Input: dimensioned drawing with shaded views. Units: mm. Origin: part minimum x, y, z. A direction names the side the tool comes from. Round coordinates to 2 decimals unless told otherwise and drop trailing zeros. Write each loop counter-clockwise with the first axis right and the second up, starting at its lowest first coordinate (ties: lowest second). Pieces come first, ordered by that corner, then holes. Notation, with made-up numbers: M 62.5,29.5 L 70.5,29.5 A31 ccw 70.5,56.5 Z; hole C 7,80.25 d10. An arc over 180 degrees is marked long. Put each result on its own line as item: value. Start each with the question number.
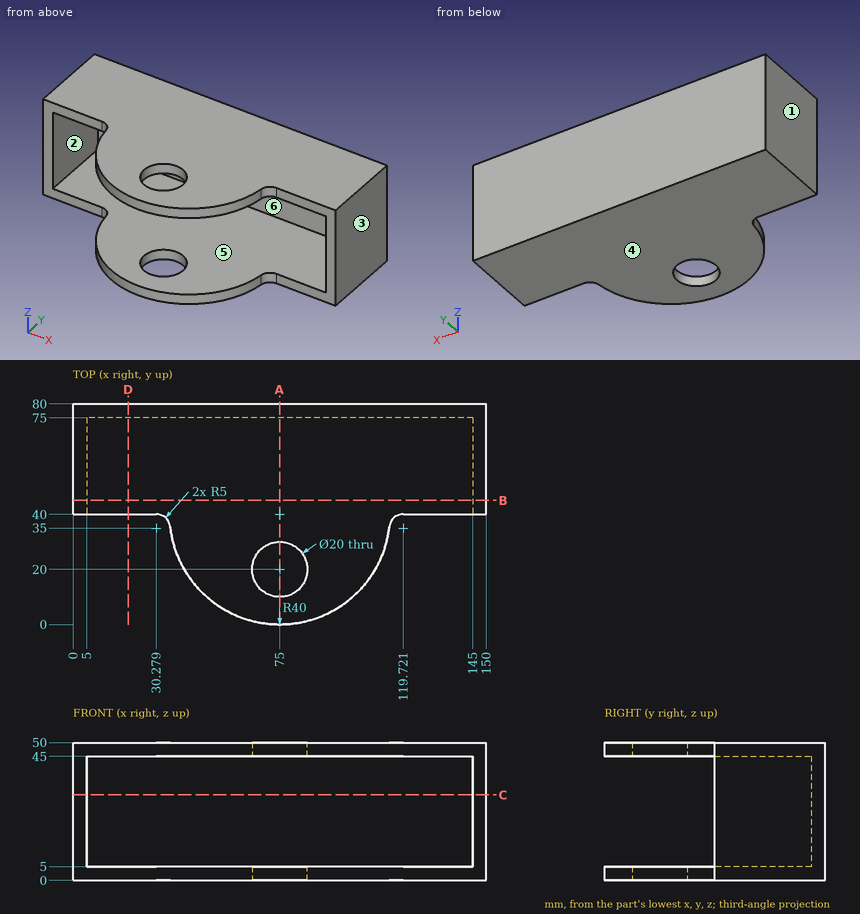
1) Access query for the marked faces 1 and 2. Directions: +Z, -Z, +X, -X, +Y, -Y. A direction counts if a zero-diameter tool reaches every point of the face in a straight line with its end or side. Return the directions, or none.
2) Section A-A, the plane x = 75. Output: boundary loops of the cut face in (y, z), and give its area (3 significant figures).
3) Section B-B, the plane y = 45. Output: boundary loops of the cut face in (x, z).
4) Section D-D, the plane x = 20. Output: boundary loops of the cut face in (y, z), and give its area (3 significant figures).
5) Ray query, probe 1 along X at (y, z) = (41, 27.5); probe 2 along Y at (x, z) = (75, 47.2); probe 3 along Z at (x, y) = (50, 51.5). Return the intervals inside material, ascending.
6) Section C-C, the plane z = 31. Output: boundary loops of the cut face in (x, y).
7) First-contact query: pin 1 (1 mm diameter, centred on x = 66, z = 31, fed in from -Y); pin 2 (23 mm diameter, centred on x = 75, y = 20, fed in from +Z); pin 3 (9 mm diameter, centred on x = 8.5, z = 27, fed in from -Y). Flat tips, straight axial feed; report the tip coordinate or a pass-through.
8) Draft query along X for the marked faces 3, 4, 5 and 6. Return one class per face: +X half, -X half, draft (parallel to the pull), parting line (faces both ways), or undercut.
Solved:
1. face 1: +Z, -Z, -X, +Y, -Y
1. face 2: -Y
2. outline: M 0,0 L 10,0 L 10,5 L 0,5 Z; M 0,45 L 10,45 L 10,50 L 0,50 Z; M 30,0 L 80,0 L 80,50 L 30,50 L 30,45 L 75,45 L 75,5 L 30,5 Z
2. area: 800 mm2
3. outline: M 0,0 L 150,0 L 150,50 L 0,50 Z; hole M 5,5 L 145,5 L 145,45 L 5,45 Z
4. outline: M 40,0 L 80,0 L 80,50 L 40,50 L 40,45 L 75,45 L 75,5 L 40,5 Z
4. area: 600 mm2
5. probe 1: x = 0 to 5, 145 to 150
5. probe 2: y = 0 to 10, 30 to 80
5. probe 3: z = 0 to 5, 45 to 50
6. outline: M 0,40 L 5,40 L 5,75 L 145,75 L 145,40 L 150,40 L 150,80 L 0,80 Z
7. pin 1: stops at y = 75
7. pin 2: stops at z = 50
7. pin 3: stops at y = 40
8. face 3: +X half
8. face 4: draft
8. face 5: undercut
8. face 6: undercut
